For this review, use the dimensioned drawing (mm, ordinates from the lowest corner) and the shaded views. Give positions to 0.01 mm unless a question says otherwise; leave off trailing zeros. Order: outer loops, then holes, each group sorted by start corner. A loop starts at its lowest first (then second) coordinate and runs counter-clockwise, first axis right, second up. Notation, with made-up numbers: (70.25, 10.5) - (81.25, 10.5) arc R10 ccw to (81.25, 21.5) - close; hole circle Ø8 at (49, 51). An arc over 180 degrees is marked (long way). Use a Markdown table: item, result. Add a question column.
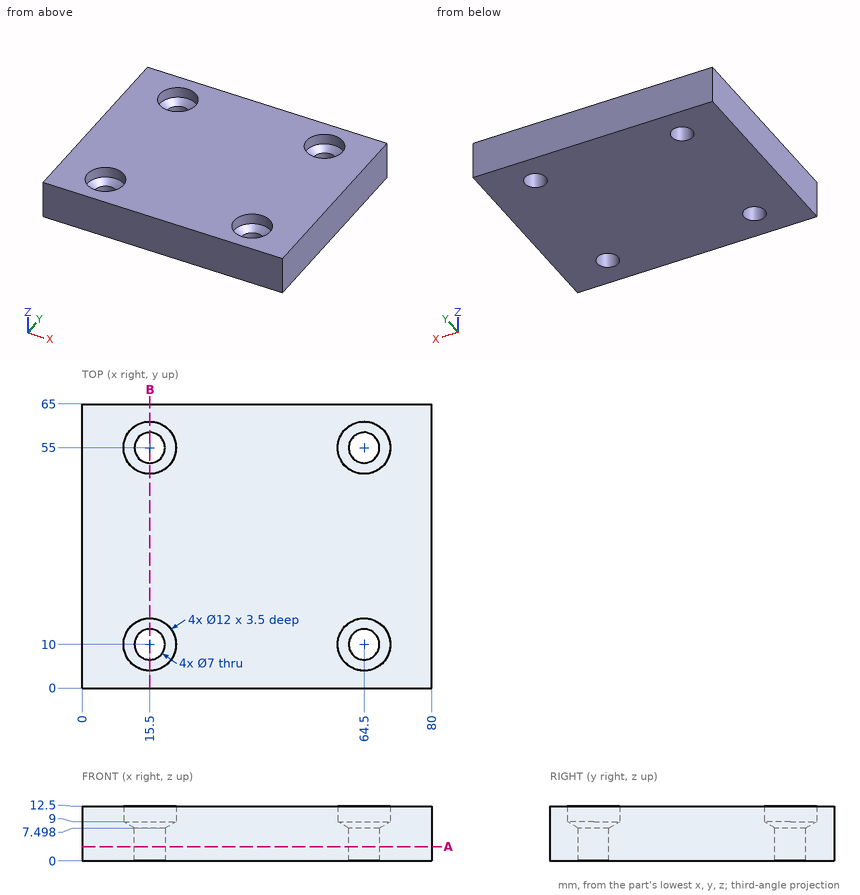
Q1. Wall thickness on probe 1 along Y at (x, z) = (15.5, 2.25); probe 2 along X at (y, z) = (5, 11.5); probe 3 along Y at (x, z) = (65.5, 5): over which ranges is each line inside the solid? List them lowest first.
Q2. We need section A-A (z = 3.25). Write out the cut boundary in (x, y), plus the area to 3 significant figures.
Q3. We need section B-B (x = 15.5). Count the separate pieces of the cut face and the enclosed holes in it, plus the area to 3 significant figures.
Here are the results:
| question | item | result |
|---|---|---|
| 1 | probe 1 | 0 to 6.5, 13.5 to 51.5, 58.5 to 65 |
| 1 | probe 2 | 0 to 12.18, 18.82 to 61.18, 67.82 to 80 |
| 1 | probe 3 | 0 to 6.65, 13.35 to 51.65, 58.35 to 65 |
| 2 | outline | (0, 0) - (80, 0) - (80, 65) - (0, 65) - close; hole circle Ø7 at (15.5, 10); hole circle Ø7 at (15.5, 55); hole circle Ø7 at (64.5, 10); hole circle Ø7 at (64.5, 55) |
| 2 | area | 5,050 mm2 |
| 3 | separate pieces | 3 |
| 3 | enclosed holes | 0 |
| 3 | area | 595 mm2 |
